Model file for the job. Use its own axes, mm. A direction names the side the tool comes from. Round coordinates to 2 decimals unless told otherwise and drop trailing zeros. Order: outer loops, then holes, each group sorted by start corner. A loop starts at its lowest first (then second) coordinate and runs counter-clockwise, first axis right, second up. Notation, with made-up numbers: M 62,-39 L 110,-39 A30 cw 110,-13 Z; hole C -9,7.25 d2. An arc over 180 degrees is marked long. Return JSON: item names as keys, results as strings. Group by question number.
Item 1: Slice it at A-A on x = 18. Write the cut outline in (y, z).
Item 2: Pull direction Z, two halves, no side cores. Call faces 3 (the face through (190, -12.5, 112)), 4 (the face through (1, -0.5, 256)), 5 (the face through (-307.51, 0.18, -68.29)): pulls with the +Z half, pulls with the -Z half, needs draft (parallel to the pull), parting line crosses it, or undercut.
Item 3: Which spindle directions (+Z, -Z, +X, -X, +Y, -Y) get a long thin tool onto all of the face, cutting with end or side? Do faces 1 (the face through (85.91, -6.58, -272.79)), 2 (the face through (-212.328, -0.175, -47.15)). Say none if no direction does.
Item 4: Pin check, flat tips, straight feed: pin 1 Ø5 at (y, z) = (9, -116) entering from -X; pin 2 Ø5 at (y, z) = (0.5, 76.5) entering from -X; pin 3 Ø6 at (x, y) = (37, -8.5) entering from -Z. Stop position of each tip, or through.
Item 5: Probe line 1 along X through (y, z) = (1.25, 0); line 2 along X through (y, z) = (-10, -19.5); line 3 along Z through (x, y) = (-160.5, -10.5). List the from-to ranges inside material, lowest first.
Item 6: Slice it at D-D on x = -225.5. Write the cut outline in (y, z).
Item 7: Slice it at B-B on z = 31. Write the cut outline in (x, y).
Item 8: Slice it at C-C on y = 3.25. Give the number of separate pieces and of enclosed holes in the cut face, then the cut area to 3 significant figures.
from build123d import *

# Parameters (mm, degrees)
SKETCH1_R           = 315
SKETCH1_R_2         = 217.5
SKETCH1_R_3         = 6
BOSS_EXTRUDE1_DEPTH = 12.5
SKETCH2_R           = 286
SKETCH2_R_2         = 255
CUT_EXTRUDE1_DEPTH  = 12


with BuildPart() as part:
    # Sketch1 → Boss-Extrude1 (new, symmetric)
    with BuildSketch(Plane(origin=(0, 0, 0), x_dir=(1, 0, 0), z_dir=(0, 1, 0))):
        with Locations(Location((0, 0, 0), (0, 0, 270))):
            Circle(SKETCH1_R)
        with Locations(Location((0, 0, 0), (0, 0, 270))):
            Circle(SKETCH1_R_2, mode=Mode.SUBTRACT)
        with Locations(Location((0, 240, 0), (0, 0, 270))):
            Circle(SKETCH1_R_3, mode=Mode.SUBTRACT)
        with Locations(Location((169.705627485, 169.705627485, 0), (0, 0, 270))):
            Circle(SKETCH1_R_3, mode=Mode.SUBTRACT)
        with Locations(Location((240, 0, 0), (0, 0, 270))):
            Circle(SKETCH1_R_3, mode=Mode.SUBTRACT)
        with Locations(Location((169.705627485, -169.705627485, 0), (0, 0, 270))):
            Circle(SKETCH1_R_3, mode=Mode.SUBTRACT)
        with Locations(Location((0, -240, 0), (0, 0, 270))):
            Circle(SKETCH1_R_3, mode=Mode.SUBTRACT)
        with Locations(Location((-169.705627485, -169.705627485, 0), (0, 0, 270))):
            Circle(SKETCH1_R_3, mode=Mode.SUBTRACT)
        with Locations(Location((-240, 0, 0), (0, 0, 270))):
            Circle(SKETCH1_R_3, mode=Mode.SUBTRACT)
        with Locations(Location((-169.705627485, 169.705627485, 0), (0, 0, 270))):
            Circle(SKETCH1_R_3, mode=Mode.SUBTRACT)
    extrude(amount=BOSS_EXTRUDE1_DEPTH, both=True)

    # Sketch2 → Cut-Extrude1 (cut)
    with BuildSketch(Plane.XZ.offset(12.5)):
        with Locations(Location((0, 0, 0), (0, 0, 270))):
            Circle(SKETCH2_R)
        with Locations(Location((0, 0, 0), (0, 0, 270))):
            Circle(SKETCH2_R_2, mode=Mode.SUBTRACT)
    extrude(amount=-CUT_EXTRUDE1_DEPTH, mode=Mode.SUBTRACT)


solid = part.part
Output values:
{
 "1": {"outline": "M -12.5,-314.49 L 12.5,-314.49 L 12.5,-216.75 L -12.5,-216.75 L -12.5,-254.36 L -0.5,-254.36 L -0.5,-285.43 L -12.5,-285.43 Z; M -12.5,216.75 L 12.5,216.75 L 12.5,314.49 L -12.5,314.49 L -12.5,285.43 L -0.5,285.43 L -0.5,254.36 L -12.5,254.36 Z"},
 "2": {"face 3": "needs draft", "face 4": "undercut", "face 5": "parting line crosses it"},
 "3": {"face 1": "-Y", "face 2": "+Y, -Y"},
 "4": {"pin 1": "x = -293.84", "pin 2": "x = -306.18", "pin 3": "z = -313.16"},
 "5": {"line 1": "-315 to -246, -234 to -217.5, 217.5 to 234, 246 to 315", "line 2": "-314.4 to -285.33, -254.25 to -216.62, 216.62 to 254.25, 285.33 to 314.4", "line 3": "-271.04 to -236.72, -198.15 to -146.79, 146.79 to 198.15, 236.72 to 271.04"},
 "6": {"outline": "M -12.5,-219.94 L 12.5,-219.94 L 12.5,219.94 L -12.5,219.94 L -12.5,175.91 L -0.5,175.91 L -0.5,119.06 L -12.5,119.06 L -12.5,-119.06 L -0.5,-119.06 L -0.5,-175.91 L -12.5,-175.91 Z"},
 "7": {"outline": "M -313.47,-12.5 L -284.31,-12.5 L -284.31,-0.5 L -253.11,-0.5 L -253.11,-12.5 L -215.28,-12.5 L -215.28,12.5 L -313.47,12.5 Z; M 215.28,-12.5 L 253.11,-12.5 L 253.11,-0.5 L 284.31,-0.5 L 284.31,-12.5 L 313.47,-12.5 L 313.47,12.5 L 215.28,12.5 Z"},
 "8": {"separate pieces": "1", "enclosed holes": "9", "area": "162,000 mm²"}
}
